Design review of the part shown in the three views and the two pictorial views. Dimensions are in mm from the part's minimum x, y and z. Round coordinates to 2 decimals unless told otherwise and drop trailing zeros. Loops run counter-clockwise (first coordinate to the right, second up) from the corner with the lowest first, then second, coordinate; pieces in that order, holes last. Notation, with made-up numbers: (-21.5, 27) -> (-12.5, 27) arc R35 ccw to (-12.5, 66) -> close; hole circle Ø2 at (70.5, 54). An arc over 180 degrees is marked (long way). Use CSV: the item, a comma, the result in double quotes. Start each with the question number.
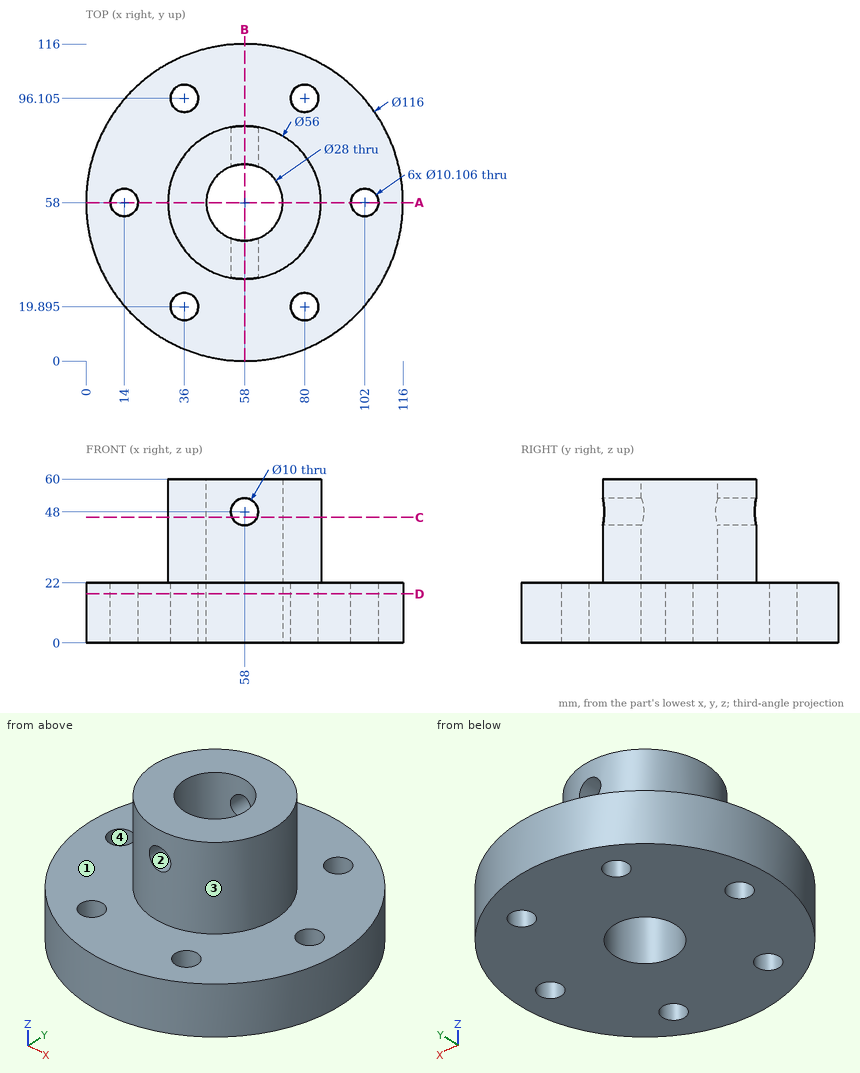
1. For line 1 along Z through (x, y) = (58, 76); line 2 along X through (y, z) = (91.5, 2.5); line 3 along Y through (x, z) = (80, 9), list the stretches that pass through material, from the lowest coordinate up. Write a range as from..to.
2. Clearance check with flat-ended pins moving along their axes: P1, Ø6, axis at x = 20, y = 62.5, coming from the +Z side; P2, Ø16, axis at x = 58, z = 48, coming from the -Y side; P3, Ø3, axis at x = 23.5, z = 24, coming from the +Y side; P4, Ø16, axis at x = 58, z = 48, coming from the +Y side. State where each tip first meets the part, or that it passes through.
3. Take a section at A-A, the plane y = 58. Give the boundary of the cut face in (x, z).
4. The part is to be moulded in two halves that separate along X. For the marked faces 1, 2, 3 and 4, say which applies: pulls with the +X half, pulls with the -X half, needs draft (parallel to the pull), parting line crosses it, or undercut.
5. Take a section at B-B, the plane x = 58. Give the boundary of the cut face in (y, z), then the cut area to 3 significant figures.
6. Take a section at C-C, the plane z = 46. Give the boundary of the cut face in (x, y).
7. Take a section at D-D, the plane z = 18. Give the boundary of the cut face in (x, y) (1 decimal).
Results:
1,line 1,"0..43, 53..60"
1,line 2,"10.65..33.92, 38.08..77.92, 82.08..105.35"
1,line 3,"4.33..14.84, 24.95..91.05, 101.16..111.67"
2,P1,"z = 22"
2,P2,"y = 30"
2,P3,"through"
2,P4,"y = 86"
3,outline,"(0, 0) -> (8.95, 0) -> (8.95, 22) -> (0, 22) -> close; (19.05, 0) -> (44, 0) -> (44, 60) -> (30, 60) -> (30, 22) -> (19.05, 22) -> close; (72, 0) -> (96.95, 0) -> (96.95, 22) -> (86, 22) -> (86, 60) -> (72, 60) -> close; (107.05, 0) -> (116, 0) -> (116, 22) -> (107.05, 22) -> close"
4,face 1,"needs draft"
4,face 2,"undercut"
4,face 3,"parting line crosses it"
4,face 4,"undercut"
5,outline,"(0, 0) -> (44, 0) -> (44, 43) -> (30, 43) -> (30, 22) -> (0, 22) -> close; (30, 53) -> (44, 53) -> (44, 60) -> (30, 60) -> close; (72, 0) -> (116, 0) -> (116, 22) -> (86, 22) -> (86, 43) -> (72, 43) -> close; (72, 53) -> (86, 53) -> (86, 60) -> (72, 60) -> close"
5,area,"2,720 mm²"
6,outline,"(53.42, 30.38) -> (53.42, 44.77) arc R14 cw to (53.42, 71.23) -> (53.42, 85.62) arc R28 ccw to start; (62.58, 30.38) arc R28 ccw to (62.58, 85.62) -> (62.58, 71.23) arc R14 cw to (62.58, 44.77) -> close"
7,outline,"circle Ø116 at (58, 58); hole circle Ø10.1 at (14, 58); hole circle Ø10.1 at (36, 19.9); hole circle Ø10.1 at (36, 96.1); hole circle Ø28 at (58, 58); hole circle Ø10.1 at (80, 19.9); hole circle Ø10.1 at (80, 96.1); hole circle Ø10.1 at (102, 58)"
